```python
from build123d import *

# Parameters (mm, degrees)
F0_W         = 26.2500010431
F0_H         = 4
F1_DEPTH     = 5
F2_W         = 19.4687498733
F2_H         = 4.5937502291
F3_DEPTH     = 43.3
F4_DEPTH     = 52.6
F5_R         = 1.3682808459
F6_DEPTH     = 25
F7_DEPTH     = 21.1
F8_T1_DEPTH  = 10
F9_T1_DEPTH  = 10
F10_T1_DEPTH = 10
F11_T1_DEPTH = 19.4687498733
F12_T1_DEPTH = 9


# Not quite as in the source:
# - a fillet or chamfer that OpenCascade refuses, or shapes differently, is made with other operations: its cross-section is extruded or revolved along the edge and cut away or added


with BuildPart() as f1:
    # F0 (on Top) → F1 (new body)
    with BuildSketch(Plane.XY):
        with Locations((-1.4218753204, -1.8281253073)):
            Rectangle(F0_W, F0_H)
    extrude(amount=F1_DEPTH)

    # F2 (on Front) → F3 (cut)
    with BuildSketch(Plane.XZ):
        with Locations((-1.7500002868, 4.375000135)):
            Rectangle(F2_W, F2_H)
    extrude(amount=F3_DEPTH, mode=Mode.SUBTRACT)

    # F2 (on Front) → F4 (cut)
    with BuildSketch(Plane.XZ):
        with Locations((-1.7500002868, 4.375000135)):
            Rectangle(F2_W, F2_H)
    extrude(amount=-F4_DEPTH, mode=Mode.SUBTRACT)

    # F5 (on Right) → F6 (cut)
    with BuildSketch(Plane.YZ):
        with Locations((-1.802527695, 3.3346994314)):
            Circle(F5_R)
    extrude(amount=-F6_DEPTH, mode=Mode.SUBTRACT)

    # F5 (on Right) → F7 (cut)
    with BuildSketch(Plane.YZ):
        with Locations((-1.802527695, 3.3346994314)):
            Circle(F5_R)
    extrude(amount=F7_DEPTH, mode=Mode.SUBTRACT)

    # F8: fillet of radius 1 on 1 edges, made by hand

    # F8_s2 → F8_t1 (cut)
    with BuildSketch(Plane.XY.offset(-2.5)):
        with BuildLine():
            ThreePointArc((10.7031252012, 0.1718746927), (11.4102319824, -0.1210185261), (11.7031252012, -0.8281253073))
            Line((11.7031252012, -0.8281253073), (11.7031252012, 0.1718746927))
            Line((11.7031252012, 0.1718746927), (10.7031252012, 0.1718746927))
        make_face()
    extrude(amount=F8_T1_DEPTH, mode=Mode.SUBTRACT)

    # F9: fillet of radius 1 on 1 edges, made by hand

    # F9_s2 → F9_t1 (cut)
    with BuildSketch(Plane.XY.offset(-2.5)):
        with BuildLine():
            ThreePointArc((-13.5468758419, 0.1718746927), (-14.2539826231, -0.1210185261), (-14.5468758419, -0.8281253073))
            Line((-14.5468758419, -0.8281253073), (-14.5468758419, 0.1718746927))
            Line((-14.5468758419, 0.1718746927), (-13.5468758419, 0.1718746927))
        make_face()
    extrude(amount=F9_T1_DEPTH, mode=Mode.SUBTRACT)

    # F10: fillet of radius 1 on 2 edges, made by hand

    # F10_s2 → F10_t1 (cut)
    with BuildSketch(Plane.XY.offset(-2.5)):
        with BuildLine():
            ThreePointArc((11.7031252012, -2.8281253073), (11.4102319824, -3.5352320885), (10.7031252012, -3.8281253073))
            Line((10.7031252012, -3.8281253073), (11.7031252012, -3.8281253073))
            Line((11.7031252012, -3.8281253073), (11.7031252012, -2.8281253073))
        make_face()
        with BuildLine():
            ThreePointArc((-13.5468758419, -3.8281253073), (-14.2539826231, -3.5352320885), (-14.5468758419, -2.8281253073))
            Line((-14.5468758419, -2.8281253073), (-14.5468758419, -3.8281253073))
            Line((-14.5468758419, -3.8281253073), (-13.5468758419, -3.8281253073))
        make_face()
    extrude(amount=F10_T1_DEPTH, mode=Mode.SUBTRACT)

    # F11: fillet of radius 5 on 2 edges, made by hand

    # F11_s2 → F11_t1 (cut)
    with BuildSketch(Plane.YZ.offset(-11.4843752235)):
        with BuildLine():
            ThreePointArc((0.1718746927, -1.4255693283), (-0.2001967002, 0.467121034), (-1.2610360303, 2.0781250205))
            Line((-1.2610360303, 2.0781250205), (0.1718746927, 2.0781250205))
            Line((0.1718746927, 2.0781250205), (0.1718746927, -1.4255693283))
        make_face()
        with BuildLine():
            ThreePointArc((-3.8281253073, -1.4769402409), (-3.4422054032, 0.4492645429), (-2.3440193596, 2.0781250205))
            Line((-2.3440193596, 2.0781250205), (-3.8281253073, 2.0781250205))
            Line((-3.8281253073, 2.0781250205), (-3.8281253073, -1.4769402409))
        make_face()
    extrude(amount=F11_T1_DEPTH, mode=Mode.SUBTRACT)

    # F12: fillet of radius 1 on 2 edges, made by hand

    # F12_s2 → F12_t1 (cut)
    with BuildSketch(Plane.XZ.offset(-2.6718746927)):
        with BuildLine():
            ThreePointArc((7.9843746498, 4), (8.2772678686, 4.7071067812), (8.9843746498, 5))
            Line((8.9843746498, 5), (7.9843746498, 5))
            Line((7.9843746498, 5), (7.9843746498, 4))
        make_face()
        with BuildLine():
            ThreePointArc((-11.4843752235, 4), (-11.7772684423, 4.7071067812), (-12.4843752235, 5))
            Line((-12.4843752235, 5), (-11.4843752235, 5))
            Line((-11.4843752235, 5), (-11.4843752235, 4))
        make_face()
    extrude(amount=F12_T1_DEPTH, mode=Mode.SUBTRACT)


solid = f1.part
```
Check sheet for the modelled part. Datum: model origin and axes. Units: mm. A direction names the side the tool comes from. Give positions to 0.01 mm unless a question says otherwise; leave off trailing zeros. Order: outer loops, then holes, each group sorted by start corner. A loop starts at its lowest first (then second) coordinate and runs counter-clockwise, first axis right, second up. Notation, with made-up numbers: M 73,40.25 L 123,40.25 A15 ccw 123,65.25 Z; hole C -20.5,-14.5 d3. An arc over 180 degrees is marked long. Answer in a Markdown table with one row per item. Add a question column.
Q1. Gauge pin test, flat ends, axial feed: pin 1 Ø0.7 at (y, z) = (-3, 3) entering from +X; pin 2 Ø1.5 at (x, y) = (5, -2.5) entering from +Z. Record the tip position at first contact, or that the pin passes through.
Q2. Access from +Z, -Z, +X, -X, +Y, -Y to the whole of each face (thin tool, end or side, straight path). Record for faces 5 (the flat face through (-11.484, 0, 2)), 6 (the flat face through (-11.484, -3, 2)), 7 (the cylindrical face through (8.55, -1.8, 4.9)), 8 (the flat face through (9, 0.172, 2)).
Q3. Release check for a two-part mould opening along X. For faces 1 (the flat face through (9, -3.828, 2)), 2 (the flat face through (-14.547, -2, 1)), 3 (the flat face through (7.984, 0, 2)), 4 (the cylindrical face through (-12.05, -1.8, 4.9)) record: released by +X, released by -X, zero draft, split by the parting line, or undercut.
Q4. Sectioned sample at A-A, the plane z = 0.7. Record the boundary of the cut face in (x, y).
Q5. Sectioned sample at B-B, the plane x = -11.75. Record the boundary of the cut face in (y, z).
Q6. Thickness scan on L1, parallel to Z at x = -7.5, y = -1.75; L2, parallel to X at y = -2.65, z = 1.9; L3, parallel to Y at x = -12.75, z = 3.55. Record the ranges inside material, lowest first.
Verdict:
| question | item | result |
|---|---|---|
| 1 | pin 1 | x = 11.69 |
| 1 | pin 2 | z = 2.08 |
| 2 | face 5 | +Z, +Y |
| 2 | face 6 | +Z, -Y |
| 2 | face 7 | +Z, +Y, -Y |
| 2 | face 8 | +Z, -Z, +X, -X, +Y |
| 3 | face 1 | zero draft |
| 3 | face 2 | released by -X |
| 3 | face 3 | undercut |
| 3 | face 4 | undercut |
| 4 | outline | M -14.55,-2.83 A1 ccw -13.55,-3.83 L -11.48,-3.83 L -11.48,-3.33 L 7.98,-3.33 L 7.98,-3.83 L 10.7,-3.83 A1 ccw 11.7,-2.83 L 11.7,-0.83 A1 ccw 10.7,0.17 L 7.98,0.17 L 7.98,-0.3 L -11.48,-0.3 L -11.48,0.17 L -13.55,0.17 A1 ccw -14.55,-0.83 Z |
| 5 | outline | M -3.83,0 L 0.17,0 L 0.17,4.68 L -1.55,4.68 A1.37 cw long -2.06,4.68 L -3.83,4.68 Z |
| 6 | L1 | 0 to 1.97 |
| 6 | L2 | -14.55 to -11.48, 7.98 to 11.7 |
| 6 | L3 | -3.83 to -3.15, -0.45 to 0.17 |
